Geometry: final body of the model. Coordinates: model frame, mm. A direction names the side the tool comes from. Coordinates: 2 decimals unless noted, no trailing zeros. Loops run counter-clockwise (first coordinate to the right, second up) from the corner with the lowest first, then second, coordinate; pieces in that order, holes last. Notation, with made-up numbers: (-6, 60.25) - (48, 60.25) arc R14 ccw to (48, 76.25) - close; hole circle Ø8 at (-14, -19). An arc over 180 degrees is marked (long way). Put each result on its own line as item: value. Start each with the question number.
1) Section D-D on x = 0.75. Output: boundary loops of the cut face in (y, z).
2) Section C-C on z = 2. Output: boundary loops of the cut face in (x, y).
3) Contact query for flat-ended pins moving along their axis: pin 1 Ø1.6 at (y, z) = (1.5, 4) entering from -X; pin 2 Ø1 at (y, z) = (2, -1.5) entering from +X; pin 3 Ø3 at (x, z) = (-2.5, 3) entering from -Y. Output: stop coordinate, or through.
4) Material intervals for line 1 along Z through (x, y) = (1.5, -2); line 2 along Y through (x, z) = (0, -5); line 3 along Y through (x, z) = (0.25, 4.25), sorted ascending. Write a range as from..to.
5) Section B-B on y = 0. Output: boundary loops of the cut face in (x, z).
6) Draft query along X for faces 1 (the flat face through (0, 0, -0.5)), 2 (the flat face through (2.4, 0, 4)), 3 (the flat face through (-1.4, -1.4, 0)). Return one class per face: +X half, -X half, draft (parallel to the pull), parting line (faces both ways), or undercut.
7) Reachability of faces 4 (the cylindrical face through (0.477, -2.146, -4.505)), 5 (the flat face through (2, 0.9, 4)), 6 (the flat face through (-0.9, -2, 4)), 7 (the flat face through (-2, -2, -0.5)) from +Z, -Z, +X, -X, +Y, -Y: full face, straight path, thin tool, end or side. Return the list, or none.
```python
from build123d import *

# Parameters (mm, degrees)
BOSS_EXTRUDE1_DEPTH = 7.9
SKETCH2_R           = 3.144549921
BOSS_EXTRUDE3_DEPTH = 0.5
SKETCH3_R           = 2.45
BOSS_EXTRUDE4_DEPTH = 7.9
SKETCH4_R           = 2.65462565
BOSS_EXTRUDE5_DEPTH = 0.3
SKETCH5_R           = 2.198604039
CUT_EXTRUDE1_DEPTH  = 7.9
CUT_EXTRUDE2_DEPTH  = 3.3
FILLET1_R           = 0.3


with BuildPart() as part:
    # Sketch1 → Boss-Extrude1 (new body)
    with BuildSketch(Plane.XY):
        Polygon((-2.4, 0.9), (-2.4, 0), (0, 0), (0, 2.4), (-0.9, 2.4), (-0.9, 0.9), align=None)
        Polygon((0, 0), (-2.4, 0), (-2.4, -0.9), (-0.9, -0.9), (-0.9, -2.4), (0, -2.4), align=None)
        Polygon((0, 2.4), (0, 0), (2.4, 0), (2.4, 0.9), (0.9, 0.9), (0.9, 2.4), align=None)
        Polygon((2.4, 0), (0, 0), (0, -2.4), (0.9, -2.4), (0.9, -0.9), (2.4, -0.9), align=None)
    extrude(amount=BOSS_EXTRUDE1_DEPTH)

    # Sketch2 → Boss-Extrude3 (add)
    with BuildSketch(Plane(origin=(0, 0, 0), x_dir=(-1, 0, 0), z_dir=(0, 0, -1))):
        Circle(SKETCH2_R)
    extrude(amount=BOSS_EXTRUDE3_DEPTH)

    # Sketch3 → Boss-Extrude4 (add)
    with BuildSketch(Plane(origin=(0, 0, -0.5), x_dir=(-1, 0, 0), z_dir=(0, 0, -1))):
        Circle(SKETCH3_R)
    extrude(amount=BOSS_EXTRUDE4_DEPTH)

    # Sketch4 → Boss-Extrude5 (add)
    with BuildSketch(Plane(origin=(0, 0, -8.4), x_dir=(-1, 0, 0), z_dir=(0, 0, -1))):
        Circle(SKETCH4_R)
    extrude(amount=-BOSS_EXTRUDE5_DEPTH)

    # Sketch5 → Cut-Extrude1 (cut)
    with BuildSketch(Plane(origin=(0, 0, -8.4), x_dir=(-1, 0, 0), z_dir=(0, 0, -1))):
        Circle(SKETCH5_R)
    extrude(amount=-CUT_EXTRUDE1_DEPTH, mode=Mode.SUBTRACT)

    # Sketch6 → Cut-Extrude2 (cut)
    with BuildSketch(Plane(origin=(0, 0, -8.4), x_dir=(-1, 0, 0), z_dir=(0, 0, -1))):
        with BuildLine():
            Line((0.375484044, 2.166303638), (0.375484044, 2.627936276))
            ThreePointArc((0.375484044, 2.627936276), (0.188215694, 2.6479449), (0, 2.65462565))
            Line((0, 2.65462565), (0, 2.198604039))
            ThreePointArc((0, 2.198604039), (0.188435389, 2.190514055), (0.375484044, 2.166303638))
        make_face()
        with BuildLine():
            Line((0, 2.198604039), (0, 2.65462565))
            ThreePointArc((0, 2.65462565), (-0.188215694, 2.6479449), (-0.375484044, 2.627936276))
            Line((-0.375484044, 2.627936276), (-0.375484044, 2.166303638))
            ThreePointArc((-0.375484044, 2.166303638), (-0.188435389, 2.190514055), (0, 2.198604039))
        make_face()
        with BuildLine():
            ThreePointArc((0, -2.65462565), (0.188215694, -2.6479449), (0.375484044, -2.627936276))
            Line((0.375484044, -2.627936276), (0.375484044, -2.166303638))
            ThreePointArc((0.375484044, -2.166303638), (0, -2.198604039), (-0.375484044, -2.166303638))
            Line((-0.375484044, -2.166303638), (-0.375484044, -2.627936276))
            ThreePointArc((-0.375484044, -2.627936276), (-0.188215694, -2.6479449), (0, -2.65462565))
        make_face()
    extrude(amount=-CUT_EXTRUDE2_DEPTH, mode=Mode.SUBTRACT)

    # Fillet1
    fillet1_edges = [part.edges().sort_by_distance(p)[0] for p in [
        (0.375484044, 2.293679776, -5.1),
        (-0.375484044, 2.293679776, -5.1),
        (-0.375484044, -2.293679776, -5.1),
        (0.375484044, -2.293679776, -5.1),
    ]]
    fillet(fillet1_edges, radius=FILLET1_R)


solid = part.part
```
Answer block:
1. outline: (-3.05, -0.5) - (-2.33, -0.5) - (-2.33, -8.1) - (-2.55, -8.1) - (-2.55, -8.4) - (-2.07, -8.4) - (-2.07, -0.5) - (2.07, -0.5) - (2.07, -8.4) - (2.55, -8.4) - (2.55, -8.1) - (2.33, -8.1) - (2.33, -0.5) - (3.05, -0.5) - (3.05, 0) - (2.4, 0) - (2.4, 7.9) - (-2.4, 7.9) - (-2.4, 0) - (-3.05, 0) - close
2. outline: (-2.4, -0.9) - (-0.9, -0.9) - (-0.9, -2.4) - (0.9, -2.4) - (0.9, -0.9) - (2.4, -0.9) - (2.4, 0.9) - (0.9, 0.9) - (0.9, 2.4) - (-0.9, 2.4) - (-0.9, 0.9) - (-2.4, 0.9) - close
3. pin 1: stops at x = -2.4
3. pin 2: stops at x = 1.94
3. pin 3: stops at y = -0.9
4. line 1: z = -8.4..-8.1, -0.5..0
4. line 2: y = -2.45..-2.2, 2.2..2.45
4. line 3: y = -2.4..2.4
5. outline: (-3.14, -0.5) - (-2.45, -0.5) - (-2.45, -8.1) - (-2.65, -8.1) - (-2.65, -8.4) - (-2.2, -8.4) - (-2.2, -0.5) - (2.2, -0.5) - (2.2, -8.4) - (2.65, -8.4) - (2.65, -8.1) - (2.45, -8.1) - (2.45, -0.5) - (3.14, -0.5) - (3.14, 0) - (2.4, 0) - (2.4, 7.9) - (-2.4, 7.9) - (-2.4, 0) - (-3.14, 0) - close
6. face 1: undercut
6. face 2: +X half
6. face 3: draft
7. face 4: -Z
7. face 5: +Z, +X, +Y
7. face 6: +Z, -X, -Y
7. face 7: none
